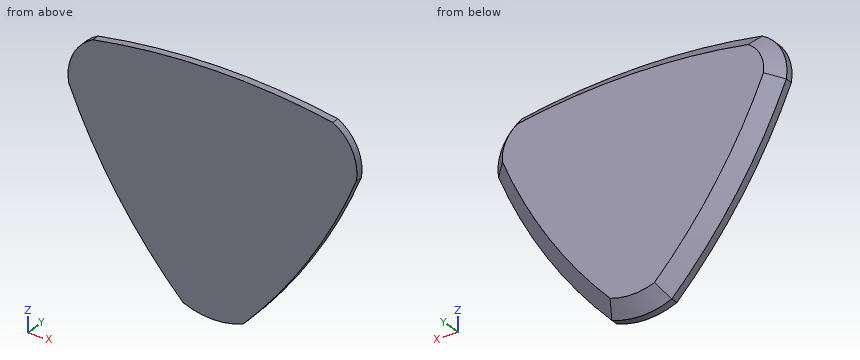
```python
from build123d import *

# Parameters (mm, degrees)
F1_DEPTH   = 11.684
F2_C1_SIZE = 7.62
F2_C2_SIZE = 7.62
F2_C3_SIZE = 7.62
F2_C4_SIZE = 7.62
F2_C5_SIZE = 7.62
F2_C6_SIZE = 7.62


with BuildPart() as f1:
    # F0 (on Front) → F1 (new body)
    with BuildSketch(Plane.XZ):
        with BuildLine():
            ThreePointArc((79.3173238635, 29.9024358392), (77.0284346929, 45.2852812744), (66.3258507848, 56.569147855))
            ThreePointArc((66.3258507848, 56.569147855), (0.0009424984, 62.4915389193), (-66.3239657879, 56.569147855))
            ThreePointArc((-66.3239657879, 56.569147855), (-77.3864565896, 45.2349353182), (-79.657331109, 29.5605547726))
            ThreePointArc((-79.657331109, 29.5605547726), (-52.5977791189, -20.9983919929), (-16.4093449712, -65.4823631048))
            ThreePointArc((-16.4093449712, -65.4823631048), (0.1379989143, -68.9400736173), (16.753109172, -65.8242329955))
            ThreePointArc((16.753109172, -65.8242329955), (52.5805254234, -20.9315825649), (79.3173238635, 29.9024358392))
        make_face()
    extrude(amount=F1_DEPTH)

    # F2: chamfer of 7.62 on 6 edges, made by hand

    # F2_c1
    f2_c1_edges = [f1.edges().sort_by_distance(p)[0] for p in [
        (0.0009424984, 0, 62.4915389193),
    ]]
    chamfer(f2_c1_edges, length=F2_C1_SIZE)

    # F2_c2
    f2_c2_edges = [f1.edges().sort_by_distance(p)[0] for p in [
        (52.5805254234, 0, -20.9315825649),
    ]]
    chamfer(f2_c2_edges, length=F2_C2_SIZE)

    # F2_c3
    f2_c3_edges = [f1.edges().sort_by_distance(p)[0] for p in [
        (-52.5977791189, 0, -20.9983919929),
    ]]
    chamfer(f2_c3_edges, length=F2_C3_SIZE)

    # F2_c4
    f2_c4_edges = [f1.edges().sort_by_distance(p)[0] for p in [
        (0.4420771354, 0, -68.9421447146),
    ]]
    chamfer(f2_c4_edges, length=F2_C4_SIZE)

    # F2_c5
    f2_c5_edges = [f1.edges().sort_by_distance(p)[0] for p in [
        (-77.0468164212, 0, 45.8983976097),
    ]]
    chamfer(f2_c5_edges, length=F2_C5_SIZE)

    # F2_c6
    f2_c6_edges = [f1.edges().sort_by_distance(p)[0] for p in [
        (76.633600388, 0, 46.0621814234),
    ]]
    chamfer(f2_c6_edges, length=F2_C6_SIZE)


solid = f1.part
```
Input: part model. Units: mm. Frame: model coordinates. Coordinates: 2 decimals unless noted, no trailing zeros. Loops run counter-clockwise (first coordinate to the right, second up) from the corner with the lowest first, then second, coordinate; pieces in that order, holes last. Notation, with made-up numbers: (-20.75, 47) - (27.25, 47) arc R24 cw to (27.25, 58) - close; hole circle Ø7 at (-17, -6.75). An arc over 180 degrees is marked (long way). Answer in a Markdown table with one row per item.
(1) Pin query (flat end, axial travel): P1, Ø3, axis at y = -10.5, z = -45.5, coming from the -X side; P2, Ø2, axis at x = -10.5, y = -3, coming from the -Z side; P3, Ø2, axis at y = -7.5, z = 12.5, coming from the +X side. Return the tip coordinate at first contact, or that it passes through.
Model answer:
| item | result |
|---|---|
| P1 | stops at x = -35.66 |
| P2 | stops at z = -63.79 |
| P3 | stops at x = 72.01 |
(2) Material intervals for L1, parallel to Z at x = 0, y = -9; L2, parallel to X at y = -9.5, z = 9; L3, parallel to X at y = -5.5, z = 28, sorted ascending. Write a range as from..to.
Model answer:
| item | result |
|---|---|
| L1 | z = -68.94..62.49 |
| L2 | x = -70.14..69.8 |
| L3 | x = -76.7..76.23 |
(3) Cut plane A-A on y = -5.5. Output: boundary loops of the cut face in (x, z), plus the area to 3 significant figures.
Model answer:
| item | result |
|---|---|
| outline | (-77.61, 30.15) arc R297.77 ccw to (-15.2, -63.69) arc R41.35 ccw to (15.55, -64.02) arc R301.65 ccw to (77.26, 30.47) arc R23.72 ccw to (65.6, 54.55) arc R372.23 ccw to (-65.62, 54.54) arc R23.46 ccw to start |
| area | 13,700 mm² |
